Part print with two shaded views. Sizes in mm from the minimum x, y, z corner. A direction names the side the tool comes from. Round coordinates to 2 decimals unless told otherwise and drop trailing zeros. Order: outer loops, then holes, each group sorted by start corner. A loop starts at its lowest first (then second) coordinate and runs counter-clockwise, first axis right, second up. Notation, with made-up numbers: M -26.75,-8.5 L 2.25,-8.5 A20 cw 2.25,4.5 Z; hole C 36,3.25 d6. An arc over 180 degrees is marked long. Answer as a JSON object with one key per item and string values.
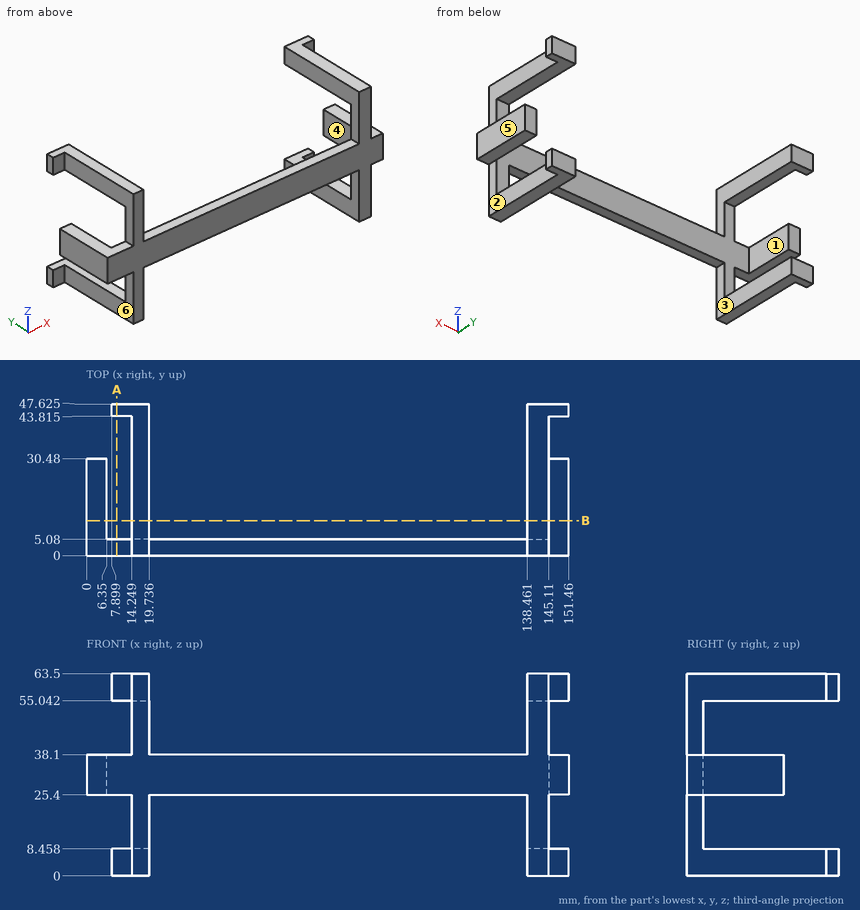
Item 1: Two-plate mould, pull along X, no slides. Class the marked faces 4, 5 and 6: released by +X, released by -X, zero draft, split by the parting line, or undercut.
Worked answers:
{"face 4": "undercut", "face 5": "released by +X", "face 6": "released by -X"}
Item 2: Saw through at A-A on x = 9.5. List the corners of the cut face in (y, z) (1 decimal).
Worked answers:
{"outline": "M 0,25.4 L 5.1,25.4 L 5.1,38.1 L 0,38.1 Z; M 43.8,0 L 47.6,0 L 47.6,8.5 L 43.8,8.5 Z; M 43.8,55 L 47.6,55 L 47.6,63.5 L 43.8,63.5 Z"}
Item 3: Saw through at B-B on y = 11. State how many separate pieces and enclosed holes the cut face has.
Worked answers:
{"separate pieces": "6", "enclosed holes": "0"}
Item 4: Wall check: line 1 along X through (y, z) = (17, 28); line 2 along Y through (x, z) = (142, 29.5); line 3 along Z through (x, y) = (108.5, 4.5). Give the ranges that are in metal, low to high. Write a range as [from, to].
Worked answers:
{"line 1": "x = [0, 6.35], [145.11, 151.46]", "line 2": "y = [0, 5.08]", "line 3": "z = [25.4, 38.1]"}
Item 5: Drop flat-ended pins along their axis: pin 1 Ø4 at (y, z) = (30.5, 10) entering from +X; pin 2 Ø5 at (x, z) = (12, 61) entering from -Y; pin 3 Ø1.5 at (x, y) = (59.5, 2.5) entering from -Z; pin 4 Ø1.9 at (x, y) = (149, 18) entering from +Z. Give the stop position or say it passes through.
Worked answers:
{"pin 1": "stops at x = 145.11", "pin 2": "stops at y = 0", "pin 3": "stops at z = 25.4", "pin 4": "stops at z = 38.1"}
Item 6: 3-axis set-ups, long thin cutter, end or side, ignore diameter. For the marked faces 1, 2 and 3: which of +Z, -Z, +X, -X, +Y, -Y reach the whole face in a straight line?
Worked answers:
{"face 1": "+Z, -Z, +Y", "face 2": "-Z, +X, -Y", "face 3": "-Z, +Y, -Y"}
